Model file for the job. Use its own axes, mm. A direction names the side the tool comes from. Round coordinates to 2 decimals unless told otherwise and drop trailing zeros. Order: outer loops, then holes, each group sorted by start corner. A loop starts at its lowest first (then second) coordinate and runs counter-clockwise, first axis right, second up. Notation, with made-up numbers: (37.5, 40.25) - (67.5, 40.25) arc R14 ccw to (67.5, 60.25) - close; hole circle Ø1 at (63, 79). An arc over 180 degrees is marked (long way). Use one line per item in the form item = value.
from build123d import *

# Parameters (mm, degrees)
CUT_EXTRUDE_2_DEPTH      = 5.5
CUT_EXTRUDE_2_DEPTH_BACK = 5.5
SKETCH_2_OUTSIDE_W       = 15.41
SKETCH_2_OUTSIDE_H       = 15.41
SKETCH_2_OUTSIDE_W_2     = 3.9
SKETCH_2_OUTSIDE_H_2     = 10
CHAMFER_2_SIZE           = 0.8
CUT_EXTRUDE_START        = -0.830011261
CUT_EXTRUDE_3_OUTLINE_R  = 2.675
CUT_EXTRUDE_3_DEPTH      = 0.830011261


# Read off the part's stored shape, not the designer's step: Вырез-Вытянуть3
with BuildPart() as part:
    # Эскиз1 → Повернуть1 (revolve)
    with BuildSketch(Plane(origin=(0, 0, 0), x_dir=(1, 0, 0), z_dir=(0, 1, 0))):
        with BuildLine():
            ThreePointArc((0, 2.9), (2.9, 0), (0, -2.9))
            Line((0, -2.9), (0, -4.5))
            ThreePointArc((0, -4.5), (4.259036435, -1.452793395), (2.75, 3.561951712))
            Line((2.75, 3.561951712), (2.75, 13.5))
            Line((2.75, 13.5), (1.5, 13.5))
            Line((1.5, 13.5), (1.5, 4.5))
            Line((1.5, 4.5), (0, 4.5))
            Line((0, 4.5), (0, 2.9))
        make_face()
    revolve(axis=Axis((0, 0, 0), (0, 0, -1)))

    # Эскиз2 outside → Вырез-Вытянуть2 (cut, two sides: drawn at the far end of the back side and taken through both)
    with BuildSketch(Plane.XY.offset(-CUT_EXTRUDE_2_DEPTH_BACK)):
        Rectangle(SKETCH_2_OUTSIDE_W, SKETCH_2_OUTSIDE_H)
        Rectangle(SKETCH_2_OUTSIDE_W_2, SKETCH_2_OUTSIDE_H_2, mode=Mode.SUBTRACT)
    extrude(amount=CUT_EXTRUDE_2_DEPTH + CUT_EXTRUDE_2_DEPTH_BACK, mode=Mode.SUBTRACT)

    # Фаска2
    chamfer_2_edges = [part.edges().sort_by_distance(p)[0] for p in [
        (1.95, 0, -5.5),
        (-1.95, 0, -5.5),
    ]]
    chamfer(chamfer_2_edges, length=CHAMFER_2_SIZE - 0.0001)  # a hair under: the kernel refuses the full size

    # Вырез-Вытянуть3 outline → Вырез-Вытянуть3 (cut)
    with BuildSketch(Plane(origin=(1.95, 0, 0), x_dir=(0, 0, -1), z_dir=(1, 0, 0)).offset(CUT_EXTRUDE_START)):
        Circle(CUT_EXTRUDE_3_OUTLINE_R)
    extrude(amount=CUT_EXTRUDE_3_DEPTH, mode=Mode.SUBTRACT)


solid = part.part
(1) Probe probe 1 along X at (y, z) = (0, -8.25); probe 2 along X at (y, z) = (-2, -3.25). List the from-to ranges inside material, lowest first. Write a range as [from, to].
Report:
probe_1 = [-2.75, -1.5], [1.5, 2.75]
probe_2 = [-1.95, 1.95]
(2) Slice it at A-A on z = -0.5. Give the cut face in (x, y), then the cut area to 3 significant figures.
Report:
outline = (-1.95, -4.02) arc R4.47 ccw to (1.95, -4.02) - (1.95, -2.63) - (1.12, -2.63) arc R2.86 cw to (-1.95, -2.09) - close; (-1.95, 2.09) arc R2.86 cw to (1.12, 2.63) - (1.95, 2.63) - (1.95, 4.02) arc R4.47 ccw to (-1.95, 4.02) - close
area = 12.9 mm2
(3) Slice it at C-C on y = 0.75. Give the cut face in (x, z).
Report:
outline = (-2.65, -13.5) - (-1.3, -13.5) - (-1.3, -4.5) - (1.3, -4.5) - (1.3, -13.5) - (2.65, -13.5) - (2.65, -5.4) - (1.95, -4.7) - (1.95, -2.57) - (1.12, -2.57) arc R2.8 cw to (-1.95, -2.01) - (-1.95, -4.7) - (-2.65, -5.4) - close; (-1.95, 2.01) arc R2.8 cw to (1.12, 2.57) - (1.95, 2.57) - (1.95, 3.99) arc R4.44 ccw to (-1.95, 3.99) - close
(4) Pull direction Z, two halves, no side cores. Call faces 1 (the face through (1.53, -2.61, 0.58)), 2 (the face through (1.2, 1.2, -13.5)), 3 (the face through (-2.747, -0.121, -8.601)): released by +Z, released by -Z, zero draft, split by the parting line, or undercut.
Report:
face_1 = undercut
face_2 = released by -Z
face_3 = zero draft
(5) Slice it at B-B on x = 0. Give the cut face in (y, z), then the cut area to 3 significant figures.
Report:
outline = (-2.75, -13.5) - (-1.5, -13.5) - (-1.5, -4.5) - (1.5, -4.5) - (1.5, -13.5) - (2.75, -13.5) - (2.75, -3.56) arc R4.5 ccw (long way) to (-2.75, -3.56) - close; hole circle Ø5.8 at (0, 0)
area = 61.3 mm2
(6) Pin check, flat tips, straight feed: pin 1 (1 mm diameter, centred on x = -1, y = -1.5, fed in from +Z); pin 2 (1.5 mm diameter, centred on x = -0.5, y = 0.5, fed in from -Z); pin 3 (2.5 mm diameter, centred on y = -2, z = -2.5, fed in from -X). Stop position of each tip, or through.
Report:
pin_1 = 4.31
pin_2 = -4.5
pin_3 = -1.95
(7) Slice it at D-D on z = 2.25. Give the cut face in (x, y).
Report:
outline = (-1.95, -3.37) arc R3.9 ccw to (1.95, -3.37) - (1.95, -1.45) - (1.12, -1.45) arc R1.83 cw (long way) to (1.12, 1.45) - (1.95, 1.45) - (1.95, 3.37) arc R3.9 ccw to (-1.95, 3.37) - close
(8) Tool access for faces 4 (the face through (1.95, -2, -2)), 5 (the face through (-1.5, -0.07, -8.94)), 6 (the face through (-1.95, -1.9, -1.4)): list every direction of +Z, -Z, +X, -X, +Y, -Y with a clear straight run to the whole face (end or side of a thin tool).
Report:
face_4 = +Z, +X, +Y, -Y
face_5 = -Z
face_6 = +Z, -X, +Y, -Y
